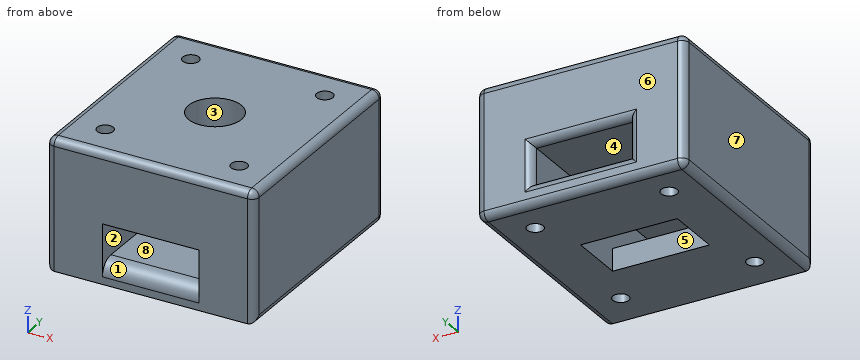
from build123d import *

# Parameters (mm, degrees)
SKETCH_W        = 28
SKETCH_H        = 17.5
SKETCH_W_2      = 13
SKETCH_H_2      = 5
PAD_DEPTH       = 30
SKETCH001_R     = 3.55
SKETCH001_R_2   = 1.075196
SKETCH001_R_3   = 1.087844
POCKET_DEPTH    = 106.725436
SKETCH002_W     = 13
SKETCH002_H     = 7.5
POCKET001_DEPTH = 5
FILLET_R        = 1
FILLET001_R     = 2


with BuildPart() as part:
    # Sketch → Pad (new body)
    with BuildSketch(Plane.XZ):
        Rectangle(SKETCH_W, SKETCH_H)
        with Locations((0, -3.25)):
            Rectangle(SKETCH_W_2, SKETCH_H_2, mode=Mode.SUBTRACT)
    extrude(amount=PAD_DEPTH)

    # Sketch001 (on DatumPlane) → Pocket (cut, through all)
    with BuildSketch(Plane(origin=(0, 0, 8.75), x_dir=(-1, 0, 0), z_dir=(0, 0, 1))):
        with Locations((0, 15)):
            Circle(SKETCH001_R)
        with Locations((9, 25)):
            Circle(SKETCH001_R_2)
        with Locations((9, 5)):
            Circle(SKETCH001_R_3)
    pocket = extrude(amount=-POCKET_DEPTH, mode=Mode.SUBTRACT)

    # Mirrored: Pocket across Sketch001 V_Axis
    add(pocket.mirror(Plane(origin=(0, 0, 8.75), x_dir=(0, 0, 1), z_dir=(-1, 0, 0))), mode=Mode.SUBTRACT)

    # Sketch002 (on Face1 of Mirrored) → Pocket001 (cut)
    with BuildSketch(Plane(origin=(0, 0, -8.75), x_dir=(1, 0, 0), z_dir=(0, 0, -1))):
        with Locations((0, 15)):
            Rectangle(SKETCH002_W, SKETCH002_H)
    extrude(amount=-POCKET001_DEPTH, mode=Mode.SUBTRACT)

    # Fillet
    fillet_edges = [part.edges().sort_by_distance(p)[0] for p in [
        (-14, -15, 8.75),
        (-14, -15, -8.75),
        (-14, 0, 0),
        (-14, -30, 0),
        (14, -15, -8.75),
        (14, -15, 8.75),
        (14, 0, 0),
        (14, -30, 0),
        (0, 0, -8.75),
        (0, 0, 8.75),
        (0, 0, -5.75),
        (6.5, 0, -3.25),
        (0, 0, -0.75),
        (-6.5, 0, -3.25),
        (0, -30, 8.75),
    ]]
    fillet(fillet_edges, radius=FILLET_R)

    # Fillet001
    fillet001_edges = [part.edges().sort_by_distance(p)[0] for p in [
        (0, -30, -5.75),
    ]]
    fillet(fillet001_edges, radius=FILLET001_R)


solid = part.part
Work out the finished part from the listing and answer in its coordinate system (mm). Face numbers are marked on the shaded views. A direction names the side the tool comes from. Round coordinates to 2 decimals unless told otherwise and drop trailing zeros. Order: outer loops, then holes, each group sorted by start corner. A loop starts at its lowest first (then second) coordinate and runs counter-clockwise, first axis right, second up. Notation, with made-up numbers: M 65,-2 L 81,-2 A21 ccw 81,15 Z; hole C -34,-32 d6. An arc over 180 degrees is marked long. Put each result on its own line as item: value. Start each with the question number.
Q1. Section B-B, the plane z = -5.25 is taken. Write down the section's boundary in (x, y), and give its area (3 significant figures).
Q2. Section D-D, the plane x = 0 is taken. Write down the section's boundary in (y, z), and give its area (3 significant figures).
Q3. A tool of negligible diameter and unlimited length cuts with its end or side. For the marked faces 1, 2, 3, 4 and 5, from which of +Z, -Z, +X, -X, +Y, -Y can it reach the whole face along a straight path? Write none if from no direction.
Q4. For a pull along X with two mould halves and no side action, classify the marked faces 6, 7 and 8 as pulls with the +X half, pulls with the -X half, needs draft (parallel to the pull), parting line crosses it, or undercut.
Q5. Straight lines are drawn through the part: L1, parallel to X at y = -5, z = -1.75; L2, parallel to X at y = -5, z = 3.5; L3, parallel to Y at x = -9, z = -1.75. For each, find the intervals that lie inside material, in ascending order. Write a range as [from, to].
Q6. Flat-ended cylindrical pins translate along their axes: pin 1 (2.5 mm diameter, centred on x = -9, y = -5, fed in from +Z); pin 2 (1.9 mm diameter, centred on x = 9, y = -25, fed in from +Z). Find the tip coordinate at first contact, or state that the pin passes through.
Q7. Section A-A, the plane y = -25 is taken. Write down the section's boundary in (x, z), and give its area (3 significant figures).
Q8. Section C-C, the plane x = 4.75 is taken. Write down the section's boundary in (y, z), and give its area (3 significant figures).
Findings below:
1. outline: M -14,-29 A1 ccw -13,-30 L -6.5,-30 L -6.5,-1 A1 ccw -7.5,0 L -13,0 A1 ccw -14,-1 Z; M 6.5,-30 L 13,-30 A1 ccw 14,-29 L 14,-1 A1 ccw 13,0 L 7.5,0 A1 ccw 6.5,-1 Z; hole C -9,-5 d2.18; hole C -9,-25 d2.15; hole C 9,-5 d2.18; hole C 9,-25 d2.15
1. area: 434 mm^2
2. outline: M -30,-8.75 L -18.75,-8.75 L -18.75,-5.75 L -28,-5.75 A2 ccw -30,-7.75 Z; M -30,-0.75 L -18.55,-0.75 L -18.55,8.75 L -29,8.75 A1 ccw -30,7.75 Z; M -11.45,-0.75 L -1,-0.75 A1 ccw 0,0.25 L 0,7.75 A1 ccw -1,8.75 L -11.45,8.75 Z; M -11.25,-8.75 L -1,-8.75 A1 ccw 0,-7.75 L 0,-6.75 A1 ccw -1,-5.75 L -11.25,-5.75 Z
2. area: 283 mm^2
3. face 1: -Y
3. face 2: none
3. face 3: +Z, -Z
3. face 4: +Y, -Y
3. face 5: -Z
4. face 6: needs draft
4. face 7: pulls with the -X half
4. face 8: undercut
5. L1: x = [-14, -10.09], [-7.91, -6.5], [6.5, 7.91], [10.09, 14]
5. L2: x = [-14, -10.09], [-7.91, 7.91], [10.09, 14]
5. L3: y = [-30, -26.08], [-23.92, -6.09], [-3.91, 0]
6. pin 1: stops at z = 8.75
6. pin 2: passes through
7. outline: M -14,-7.75 A1 ccw -13,-8.75 L -10.08,-8.75 L -10.08,8.75 L -13,8.75 A1 ccw -14,7.75 Z; M -7.92,-8.75 L 7.92,-8.75 L 7.92,8.75 L -7.92,8.75 Z; M 10.08,-8.75 L 13,-8.75 A1 ccw 14,-7.75 L 14,7.75 A1 ccw 13,8.75 L 10.08,8.75 Z; hole M -6.5,-5.75 L 6.5,-5.75 L 6.5,-0.75 L -6.5,-0.75 Z
7. area: 349 mm^2
8. outline: M -30,-8.75 L -18.75,-8.75 L -18.75,-5.75 L -28,-5.75 A2 ccw -30,-7.75 Z; M -30,-0.75 L -1,-0.75 A1 ccw 0,0.25 L 0,7.75 A1 ccw -1,8.75 L -29,8.75 A1 ccw -30,7.75 Z; M -11.25,-8.75 L -1,-8.75 A1 ccw 0,-7.75 L 0,-6.75 A1 ccw -1,-5.75 L -11.25,-5.75 Z
8. area: 351 mm^2
